Print and shaded views of the part. All mm, measured from the part's lowest x, y and z. A direction names the side the tool comes from. Round coordinates to 2 decimals unless told otherwise and drop trailing zeros. Loops run counter-clockwise (first coordinate to the right, second up) from the corner with the lowest first, then second, coordinate; pieces in that order, holes last. Notation, with made-up numbers: (-9.75, -13) - (37.25, -13) arc R19 cw to (37.25, 24) - close; hole circle Ø7 at (9.25, 15.25). An arc over 180 degrees is marked (long way). Use one line per item in the form item = value.
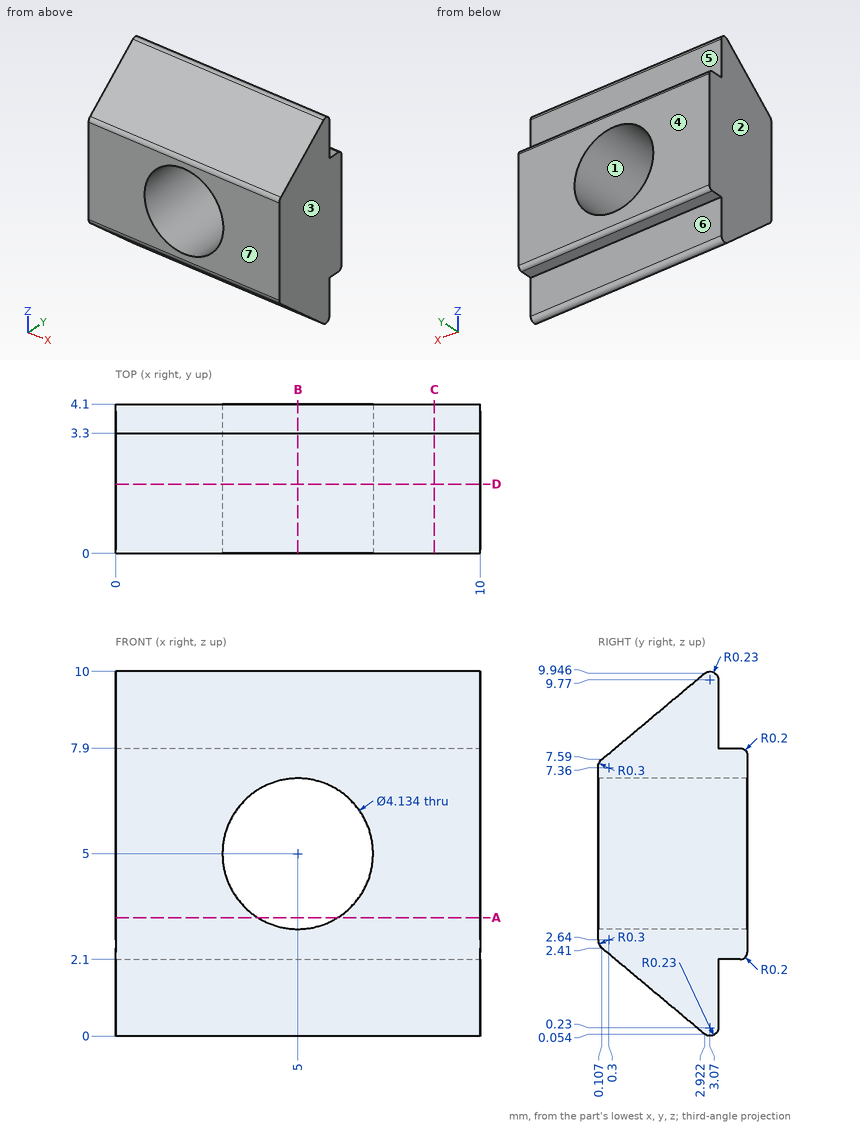
1) Slice it at A-A (z = 3.25). Write the cut outline in (x, y).
Report:
outline = (0, 0) - (3.9, 0) - (3.9, 4.1) - (0, 4.1) - close; (6.1, 0) - (10, 0) - (10, 4.1) - (6.1, 4.1) - close
2) Tool access for the marked faces 5, 6 and 7: list every direction of +Z, -Z, +X, -X, +Y, -Y with a clear straight run to the whole face (end or side of a thin tool).
Report:
face_5 = +Z, +X, -X, +Y
face_6 = -Z, +X, -X, +Y
face_7 = +Z, -Z, +X, -X, -Y
3) Drill centre lines: probe 1 along Z at (x, y) = (6.5, 1) (1 decimal); probe 2 along Z at (x, y) = (6, 3.85); probe 3 along Z at (x, y) = (0.75, 3.1). Where is each one in solid material? Low to high.
Report:
probe_1 = 1.7 to 3.6, 6.4 to 8.3
probe_2 = 2.1 to 3.19, 6.81 to 7.9
probe_3 = 0 to 10
4) Two-plate mould, pull along X, no slides. Class the marked faces 1, 2, 3 and 4: +X half, -X half, draft (parallel to the pull), parting line (faces both ways), or undercut.
Report:
face_1 = undercut
face_2 = -X half
face_3 = +X half
face_4 = draft
5) Slice it at D-D (y = 1.9). Write the cut outline in (x, z).
Report:
outline = (0, 0.91) - (10, 0.91) - (10, 9.09) - (0, 9.09) - close; hole circle Ø4.13 at (5, 5)
6) Slice it at B-B (x = 5). Write the cut outline in (y, z).
Report:
outline = (0, 2.64) arc R0.3 ccw to (0.11, 2.41) - (2.92, 0.05) arc R0.23 ccw to (3.3, 0.23) - (3.3, 2.1) - (3.9, 2.1) arc R0.2 ccw to (4.1, 2.3) - (4.1, 2.93) - (0, 2.93) - close; (0, 7.07) - (4.1, 7.07) - (4.1, 7.7) arc R0.2 ccw to (3.9, 7.9) - (3.3, 7.9) - (3.3, 9.77) arc R0.23 ccw to (2.92, 9.95) - (0.11, 7.59) arc R0.3 ccw to (0, 7.36) - close
7) Slice it at C-C (x = 8.75). Write the cut outline in (y, z).
Report:
outline = (0, 2.64) arc R0.3 ccw to (0.11, 2.41) - (2.92, 0.05) arc R0.23 ccw to (3.3, 0.23) - (3.3, 2.1) - (3.9, 2.1) arc R0.2 ccw to (4.1, 2.3) - (4.1, 7.7) arc R0.2 ccw to (3.9, 7.9) - (3.3, 7.9) - (3.3, 9.77) arc R0.23 ccw to (2.92, 9.95) - (0.11, 7.59) arc R0.3 ccw to (0, 7.36) - close
8) Flat gauge pins, fed straight in: pin 1 (0.6 mm diameter, centred on x = 3.5, z = 9, fed in from +Y); pin 2 (0.7 mm diameter, centred on x = 5, y = 3.5, fed in from -Z) (1 decimal); pin 3 (3 mm diameter, centred on x = 4.5, z = 1, fed in from -Y) (1 decimal). Where does each tip first touch, or does it go through?
Report:
pin_1 = 3.3
pin_2 = 0
pin_3 = 0
